Part model, mm, in its own coordinate system. Face numbers are marked on the shaded views. Round coordinates to 2 decimals unless told otherwise and drop trailing zeros. Write each loop counter-clockwise with the first axis right and the second up, starting at its lowest first coordinate (ties: lowest second). Pieces come first, ordered by that corner, then holes. Notation, with made-up numbers: M -31,73.25 L -10,73.25 A7 ccw -10,79.25 Z; hole C 44,-0.75 d3. An arc over 180 degrees is marked long. Answer as a JSON object with one key per item and string values. Group by question number.
1. Two-plate mould, pull along Y, no slides. Class the marked faces 1 and 2: +Y half, -Y half, draft (parallel to the pull), parting line (faces both ways), or undercut.
2. Band-saw the part on A-A, the plane z = 0. Write the cut outline in (x, y), plus the area to 3 significant figures.
3. Band-saw the part on D-D, the plane z = 39. Write the cut outline in (x, y), plus the area to 3 significant figures.
4. Band-saw the part on C-C, the plane x = 0. Write the cut outline in (y, z).
5. Band-saw the part on B-B, the plane y = 0.3. Write the cut outline in (x, z).
6. Drop flat-ended pins along their axis: pin 1 (2.5 mm diameter, centred on x = 0, z = 39, fed in from +Y) (3 decimals); pin 2 (0.6 mm diameter, centred on x = 9.5, y = 1, fed in from +Z); pin 3 (0.6 mm diameter, centred on y = 0.5, z = -40, fed in from +X); pin 4 (4 mm diameter, centred on x = 39, z = 0, fed in from +Y). Give the stop position or say it passes through.
7. Drill centre lines: line 1 (X direction, y = 1.2, z = 0); line 2 (Z direction, x = 0, y = 0.7); line 3 (X direction, y = 1.8, z = 0.5). Where is each one in solid material? Low to high. Write a range as from..to.
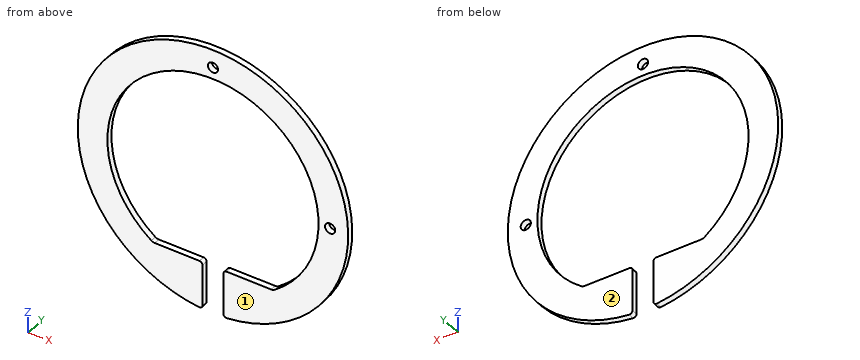
from build123d import *

# Parameters (mm, degrees)
BOSS_EXTRU_1_DEPTH      = 2
ESQUISSE2_R             = 1.7
ENL_V_MAT_EXTRU_1_DEPTH = 3
CONG_1_R                = 1
CONG_2_R                = 2


with BuildPart() as part:
    # Esquisse1 → Boss.-Extru.1 (new body)
    with BuildSketch(Plane(origin=(0, 0, 0), x_dir=(1, 0, 0), z_dir=(0, 1, 0))):
        with BuildLine():
            Line((-3.5, 28.89), (-3.5, 44.863682417))
            ThreePointArc((-3.5, 44.863682417), (0, -45), (3.5, 44.863682417))
            Line((3.5, 44.863682417), (3.5, 28.89))
            Line((3.5, 28.89), (20, 28.89))
            ThreePointArc((20, 28.89), (0, -35.137331999), (-20, 28.89))
            Line((-20, 28.89), (-3.5, 28.89))
        make_face()
    extrude(amount=BOSS_EXTRU_1_DEPTH)

    # Esquisse2 → Enlèv. mat.-Extru.1 (cut, through all)
    with BuildSketch(Plane(origin=(0, 2, 0), x_dir=(1, 0, 0), z_dir=(0, 1, 0))):
        with Locations((39, 0)):
            Circle(ESQUISSE2_R)
        with Locations((0, -39)):
            Circle(ESQUISSE2_R)
    extrude(amount=-ENL_V_MAT_EXTRU_1_DEPTH, mode=Mode.SUBTRACT)

    # Congé1
    cong_1_edges = [part.edges().sort_by_distance(p)[0] for p in [
        (-3.5, 1, -44.863682417),
        (-3.5, 1, -28.89),
        (3.5, 1, -28.89),
        (3.5, 1, -44.863682417),
    ]]
    fillet(cong_1_edges, radius=CONG_1_R)

    # Congé2
    cong_2_edges = [part.edges().sort_by_distance(p)[0] for p in [
        (-20, 1, -28.89),
        (20, 1, -28.89),
    ]]
    fillet(cong_2_edges, radius=CONG_2_R)


solid = part.part
Worked answers:
{
 "1": {"face 1": "-Y half", "face 2": "+Y half"},
 "2": {"outline": "M -45,0 L -35.14,0 L -35.14,2 L -45,2 Z; M 35.14,0 L 37.3,0 L 37.3,2 L 35.14,2 Z; M 40.7,0 L 45,0 L 45,2 L 40.7,2 Z", "area": "32.7 mm^2"},
 "3": {"outline": "M -22.45,0 L -1.7,0 L -1.7,2 L -22.45,2 Z; M 1.7,0 L 22.45,0 L 22.45,2 L 1.7,2 Z", "area": "83.0 mm^2"},
 "4": {"outline": "M 0,35.14 L 2,35.14 L 2,37.3 L 0,37.3 Z; M 0,40.7 L 2,40.7 L 2,45 L 0,45 Z"},
 "5": {"outline": "M -20.53,-28.51 A35.14 cw long 20.53,-28.51 A2 cw 19.37,-28.89 L 4.5,-28.89 A1 ccw 3.5,-29.89 L 3.5,-43.77 A1 ccw 4.6,-44.76 A45 ccw long -4.6,-44.76 A1 ccw -3.5,-43.77 L -3.5,-29.89 A1 ccw -4.5,-28.89 L -19.37,-28.89 A2 cw Z; hole C 0,39 d3.4; hole C 39,0 d3.4"},
 "6": {"pin 1": "passes through", "pin 2": "stops at z = 44.05", "pin 3": "stops at x = 21.19", "pin 4": "stops at y = 2"},
 "7": {"line 1": "x = -45..-35.14, 35.14..37.3, 40.7..45", "line 2": "z = 35.14..37.3, 40.7..45", "line 3": "x = -45..-35.13, 35.13..37.38, 40.62..45"}
}
